from build123d import *

# Parameters (mm, degrees)
SKETCH1_W               = 19
SKETCH1_H               = 29
SKETCH1_R               = 2.5
BOSS_EXTRUDE2_DEPTH     = 1
SKETCH3_R               = 3
SKETCH3_R_2             = 2.5
SKETCH3_RX              = 0.922092895
SKETCH3_RY              = 0.713508325
SKETCH3_R_3             = 0.45
BOSS_EXTRUDE3_DEPTH     = 0.25
SKETCH4_R               = 0.45
CUT_EXTRUDE1_DEPTH      = 1.25
CUT_EXTRUDE1_DEPTH_BACK = 2
SKETCH5_W               = 12
SKETCH5_H               = 15.5
BOSS_EXTRUDE4_DEPTH     = 5.5
SKETCH7_W               = 1.5
SKETCH7_H               = 1.5
SKETCH7_W_2             = 0.75
CUT_EXTRUDE2_DEPTH      = 6


with BuildPart() as part:
    # Sketch1 → Boss-Extrude2 (new body)
    with BuildSketch(Plane(origin=(0, 0, 0), x_dir=(1, 0, 0), z_dir=(0, 1, 0))):
        Rectangle(SKETCH1_W, SKETCH1_H)
        with Locations((0, -7.5)):
            Circle(SKETCH1_R, mode=Mode.SUBTRACT)
    extrude(amount=-BOSS_EXTRUDE2_DEPTH)

    # Sketch3 → Boss-Extrude3 (add)
    with BuildSketch(Plane(origin=(0, 0, 0), x_dir=(1, 0, 0), z_dir=(0, 1, 0))):
        with Locations((0, -7.5)):
            Circle(SKETCH3_R)
        with Locations((0, -7.5)):
            Circle(SKETCH3_R_2, mode=Mode.SUBTRACT)
        with Locations(Location((0, -13), (0, 0, -90))):
            Ellipse(SKETCH3_RX, SKETCH3_RY)
        with Locations((0, -13)):
            Circle(SKETCH3_R_3, mode=Mode.SUBTRACT)
        with Locations(Location((2.54, -13), (0, 0, -90))):
            Ellipse(SKETCH3_RX, SKETCH3_RY)
        with Locations((2.54, -13)):
            Circle(SKETCH3_R_3, mode=Mode.SUBTRACT)
        with Locations(Location((-2.54, -13), (0, 0, -90))):
            Ellipse(SKETCH3_RX, SKETCH3_RY)
        with Locations((-2.54, -13)):
            Circle(SKETCH3_R_3, mode=Mode.SUBTRACT)
    extrude(amount=BOSS_EXTRUDE3_DEPTH)

    # Sketch4 → Cut-Extrude1 (cut, two sides)
    with BuildSketch(Plane(origin=(0, 0, 0), x_dir=(1, 0, 0), z_dir=(0, 1, 0))) as cut_extrude1_sk:
        with Locations((-2.54, -13)):
            Circle(SKETCH4_R)
        with Locations((0, -13)):
            Circle(SKETCH4_R)
        with Locations((2.54, -13)):
            Circle(SKETCH4_R)
    extrude(amount=CUT_EXTRUDE1_DEPTH, mode=Mode.SUBTRACT)
    extrude(cut_extrude1_sk.sketch, amount=-CUT_EXTRUDE1_DEPTH_BACK, mode=Mode.SUBTRACT)

    # Sketch5 → Boss-Extrude4 (add)
    with BuildSketch(Plane(origin=(0, 0, 0), x_dir=(1, 0, 0), z_dir=(0, 1, 0))):
        with Locations((0, 5.065615618)):
            Rectangle(SKETCH5_W, SKETCH5_H)
    extrude(amount=BOSS_EXTRUDE4_DEPTH)

    # Sketch7 → Cut-Extrude2 (cut)
    with BuildSketch(Plane(origin=(0, 0, 0), x_dir=(1, 0, 0), z_dir=(0, 1, 0))):
        with Locations((-3, 12.050904241)):
            Rectangle(SKETCH7_W, SKETCH7_H)
        with Locations((0, 12.050904241)):
            Rectangle(SKETCH7_W, SKETCH7_H)
        with Locations((3, 12.050904241)):
            Rectangle(SKETCH7_W, SKETCH7_H)
        with Locations((-3, 9.080326995)):
            Rectangle(SKETCH7_W, SKETCH7_H)
        with Locations((3, 9.080326995)):
            Rectangle(SKETCH7_W, SKETCH7_H)
        with Locations((0, 9.080326995)):
            Rectangle(SKETCH7_W, SKETCH7_H)
        with Locations((-3, 6.080326995)):
            Rectangle(SKETCH7_W, SKETCH7_H)
        with Locations((0, 6.080326995)):
            Rectangle(SKETCH7_W, SKETCH7_H)
        with Locations((3, 6.080326995)):
            Rectangle(SKETCH7_W, SKETCH7_H)
        with Locations((-3, 3.080326995)):
            Rectangle(SKETCH7_W, SKETCH7_H)
        with Locations((3, 3.080326995)):
            Rectangle(SKETCH7_W, SKETCH7_H)
        with Locations((0, 3.080326995)):
            Rectangle(SKETCH7_W, SKETCH7_H)
        with Locations((-3, 0.080326995)):
            Rectangle(SKETCH7_W, SKETCH7_H)
        with Locations((0, 0.080326995)):
            Rectangle(SKETCH7_W, SKETCH7_H)
        with Locations((3, 0.080326995)):
            Rectangle(SKETCH7_W, SKETCH7_H)
        with Locations((5.625, 6.080326995)):
            Rectangle(SKETCH7_W_2, SKETCH7_H)
        with Locations((-5.625, 6.080326995)):
            Rectangle(SKETCH7_W_2, SKETCH7_H)
        with Locations((5.625, 9.080326995)):
            Rectangle(SKETCH7_W_2, SKETCH7_H)
        with Locations((-5.625, 9.080326995)):
            Rectangle(SKETCH7_W_2, SKETCH7_H)
        with Locations((5.625, 0.080326995)):
            Rectangle(SKETCH7_W_2, SKETCH7_H)
        with Locations((-5.625, 0.080326995)):
            Rectangle(SKETCH7_W_2, SKETCH7_H)
    extrude(amount=CUT_EXTRUDE2_DEPTH, mode=Mode.SUBTRACT)


solid = part.part
Work out the finished part from the listing and answer in its coordinate system (mm). A direction names the side the tool comes from. Round coordinates to 2 decimals unless told otherwise and drop trailing zeros. Order: outer loops, then holes, each group sorted by start corner. A loop starts at its lowest first (then second) coordinate and runs counter-clockwise, first axis right, second up. Notation, with made-up numbers: M 12.5,34 L 62.5,34 A16 ccw 62.5,48 Z; hole C 21,43 d11. An arc over 180 degrees is marked long. Put each result on its own line as item: value. Start each with the question number.
Q1. Straight lines are drawn through the part: L1, parallel to Z at x = 5.75, y = 1.25; L2, parallel to X at y = -0.4, z = 13; L3, parallel to X at y = 1, z = -6.5. For each, find the intervals that lie inside material, in ascending order. Write a range as [from, to].
Q2. A tool of negligible diameter and unlimited length cuts with its end or side. For faces 4 (the flat face through (6, 3, -8)), 5 (the flat face through (5.25, 3, 0)), 6 (the flat face through (-3, 0, -3)), from which of +Z, -Z, +X, -X, +Y, -Y can it reach the whole face along a straight path? Write none if from no direction.
Q3. Section C-C, the plane z = -0.5 is taken. Write down the section's boundary in (x, y).
Q4. For a pull along X with two mould halves and no side action, classify faces 1 (the flat face through (5.25, 3, -6)), 2 (the flat face through (-5.25, 3, -6)), 3 (the flat face through (3, 3, -2.33)) as pulls with the +X half, pulls with the -X half, needs draft (parallel to the pull), parting line crosses it, or undercut.
Q5. Section A-A, the plane y = -0.5 is taken. Write down the section's boundary in (x, z), and give its area (3 significant figures).
Q6. Section B-B, the plane z = 7.5 is taken. Write down the section's boundary in (x, y).
Q7. Flat-ended cylindrical pins translate along their axes: pin 1 (1.2 mm diameter, centred on y = 2, z = 0, fed in from +X); pin 2 (1.2 mm diameter, centred on y = 1.5, z = -9.5, fed in from -X); pin 3 (0.8 mm diameter, centred on y = 3, z = -3, fed in from +X). Find the tip coordinate at first contact, or state that the pin passes through.
Q8. Section D-D, the plane x = 0 is taken. Give the number of separate pieces and of enclosed holes in the cut face, and give its area (3 significant figures).
Findings below:
1. L1: z = [-12.82, -9.83], [-8.33, -6.83], [-5.33, -0.83], [0.67, 2.68]
1. L2: x = [-9.5, -2.99], [-2.09, -0.45], [0.45, 2.09], [2.99, 9.5]
1. L3: x = [-5.25, -3.75], [-2.25, -0.75], [0.75, 2.25], [3.75, 5.25]
2. face 4: +Z, -Z, +X, +Y
2. face 5: +X, +Y
2. face 6: +Y
3. outline: M -9.5,-1 L 9.5,-1 L 9.5,0 L 5.25,0 L 5.25,5.5 L 3.75,5.5 L 3.75,0 L 2.25,0 L 2.25,5.5 L 0.75,5.5 L 0.75,0 L -0.75,0 L -0.75,5.5 L -2.25,5.5 L -2.25,0 L -3.75,0 L -3.75,5.5 L -5.25,5.5 L -5.25,0 L -9.5,0 Z
4. face 1: pulls with the +X half
4. face 2: pulls with the -X half
4. face 3: undercut
5. outline: M -9.5,-14.5 L 9.5,-14.5 L 9.5,14.5 L -9.5,14.5 Z; hole C -2.54,13 d0.9; hole C 0,7.5 d5; hole C 0,13 d0.9; hole C 2.54,13 d0.9
5. area: 529 mm^2
6. outline: M -9.5,-1 L -2.5,-1 L -2.5,0.25 L -3,0.25 L -3,0 L -9.5,0 Z; M 2.5,-1 L 9.5,-1 L 9.5,0 L 3,0 L 3,0.25 L 2.5,0.25 Z
7. pin 1: stops at x = 5.25
7. pin 2: stops at x = -6
7. pin 3: stops at x = 6
8. separate pieces: 3
8. enclosed holes: 0
8. area: 67.6 mm^2
